Geometry: final body of the model. Coordinates: model frame, mm. A direction names the side the tool comes from. Round coordinates to 2 decimals unless told otherwise and drop trailing zeros. Loops run counter-clockwise (first coordinate to the right, second up) from the corner with the lowest first, then second, coordinate; pieces in that order, holes last. Notation, with made-up numbers: (29, 48) - (55, 48) arc R20 ccw to (55, 57) - close; hole circle Ø8 at (-23, 72). An arc over 180 degrees is marked (long way). Answer as a JSON object with one key per item and string values. Group by question number.
Item 1: Line query: line 1 (Y direction, x = 2.5, z = 1.4) (3 decimals); line 2 (Y direction, x = 20, z = 4.25) (3 decimals); line 3 (Z direction, x = 20.75, y = -14.5) (3 decimals). Output: solid intervals per line, ascending.
Item 2: Draft query along Z for faces 1 (the face through (9.774, -10.742, 1.565)), 2 (the face through (22.7, -21.57, 11.89)), 3 (the face through (15.72, -21.61, 10.09)), 4 (the face through (6.86, -21.61, 10.24)). Return one class per face: released by +Z, released by -Z, zero draft, split by the parting line, or undercut.
Item 3: Section D-D (y = -10). Return the cut outline in (x, z) (3 decimals), plus the area to 3 significant figures.
Item 4: Reachability of faces 5 (the face through (11, -20, 8)), 6 (the face through (11, -23.175, 7)) from +Z, -Z, +X, -X, +Y, -Y: full face, straight path, thin tool, end or side. Return the list, or none.
Item 5: Section C-C (y = -2). Return the cut outline in (x, z) (3 decimals).
Item 6: Section B-B (x = 11.5). Return the cut outline in (y, z) (3 decimals), plus the area to 3 significant figures.
Item 7: Section A-A (x = 2.5). Return the cut outline in (y, z) (3 decimals).
Item 8: First-contact query: pin 1 (3 mm diameter, centred on y = -17, z = 4.5, fed in from -X); pin 2 (4 mm diameter, centred on x = 20.5, y = -2, fed in from +Z) (3 decimals); pin 3 (5 mm diameter, centred on y = 1.5, z = 7.5, fed in from -X); pin 4 (4.5 mm diameter, centred on x = 6.48, z = 8.56, fed in from +Y). Flat tips, straight axial feed; report the tip coordinate or a pass-through.
```python
from build123d import *

# Parameters (mm, degrees)
SKETCH1_W             = 23
SKETCH1_H             = 38.970207686
SKETCH1_R             = 1.7272
SKETCH1_R_2           = 1.4732
BOSS_EXTRUDE1_DEPTH   = 3.175
BOSS_EXTRUDE2_START   = 3.175
SKETCH1_3_W           = 23
SKETCH1_3_H           = 3.175
BOSS_EXTRUDE2_DEPTH   = 9
F_8_32_TAPPED_HOLE1_D = 3.4544
FILLET1_R             = 1


with BuildPart() as part:
    # Sketch1 → Boss-Extrude1 (new body)
    with BuildSketch(Plane.XY):
        with Locations((11.5, -3.689896157)):
            Rectangle(SKETCH1_W, SKETCH1_H)
        with Locations((11.5, -10.81790431)):
            Circle(SKETCH1_R, mode=Mode.SUBTRACT)
        with Locations((2.5, -2)):
            Circle(SKETCH1_R_2, mode=Mode.SUBTRACT)
        with Locations((20.5, -2)):
            Circle(SKETCH1_R_2, mode=Mode.SUBTRACT)
        with Locations((11.5, 7.18209569)):
            Circle(SKETCH1_R, mode=Mode.SUBTRACT)
    extrude(amount=BOSS_EXTRUDE1_DEPTH)

    # Sketch1<3> → Boss-Extrude2 (add)
    with BuildSketch(Plane.XY.offset(BOSS_EXTRUDE2_START)):
        with Locations((11.5, -21.5875)):
            Rectangle(SKETCH1_3_W, SKETCH1_3_H)
    extrude(amount=BOSS_EXTRUDE2_DEPTH)

    # #8-32 Tapped Hole1 (through all)
    with Locations(Plane(origin=(6.4835, -20, 8.5555), x_dir=(1, 0, 0), z_dir=(0, 1, 0))):
        with Locations((0, 0), (10.033, 0)):
            Hole(F_8_32_TAPPED_HOLE1_D / 2)

    # Fillet1
    fillet1_edges = [part.edges().sort_by_distance(p)[0] for p in [
        (11.5, -23.175, 0),
        (0, -21.5875, 12.175),
        (11.5, -20, 3.175),
        (23, -21.5875, 12.175),
    ]]
    fillet(fillet1_edges, radius=FILLET1_R)


solid = part.part
```
Values:
{
 "1": {"line 1": "y = -23.175 to -3.473, -0.527 to 15.795", "line 2": "y = -23.175 to -20", "line 3": "z = 0 to 3.175"},
 "2": {"face 1": "zero draft", "face 2": "released by +Z", "face 3": "undercut", "face 4": "undercut"},
 "3": {"outline": "(0, 0) - (9.979, 0) - (9.979, 3.175) - (0, 3.175) - close; (13.021, 0) - (23, 0) - (23, 3.175) - (13.021, 3.175) - close", "area": "63.4 mm^2"},
 "4": {"face 5": "+Z, +X, -X, +Y", "face 6": "+Z, -Z, +X, -X, -Y"},
 "5": {"outline": "(0, 0) - (1.027, 0) - (1.027, 3.175) - (0, 3.175) - close; (3.973, 0) - (19.027, 0) - (19.027, 3.175) - (3.973, 3.175) - close; (21.973, 0) - (23, 0) - (23, 3.175) - (21.973, 3.175) - close"},
 "6": {"outline": "(-23.175, 1) arc R1 ccw to (-22.175, 0) - (-12.545, 0) - (-12.545, 3.175) - (-19, 3.175) arc R1 cw to (-20, 4.175) - (-20, 12.175) - (-23.175, 12.175) - close; (-9.091, 0) - (5.455, 0) - (5.455, 3.175) - (-9.091, 3.175) - close; (8.909, 0) - (15.795, 0) - (15.795, 3.175) - (8.909, 3.175) - close", "area": "130 mm^2"},
 "7": {"outline": "(-23.175, 1) arc R1 ccw to (-22.175, 0) - (-3.473, 0) - (-3.473, 3.175) - (-19, 3.175) arc R1 cw to (-20, 4.175) - (-20, 12.175) - (-23.175, 12.175) - close; (-0.527, 0) - (15.795, 0) - (15.795, 3.175) - (-0.527, 3.175) - close"},
 "8": {"pin 1": "stops at x = 0", "pin 2": "stops at z = 3.175", "pin 3": "passes through", "pin 4": "stops at y = -20"}
}
